Can you work these out from the model? Positions are in its coordinate system, mm. A direction names the side the tool comes from. Give positions to 0.01 mm unless a question says otherwise; leave off trailing zeros. Loops run counter-clockwise (first coordinate to the right, second up) from the corner with the lowest first, then second, coordinate; pieces in that order, holes last. Notation, with made-up numbers: (2.5, 51) - (42.5, 51) arc R13 ccw to (42.5, 73) - close; hole circle Ø8 at (13, 68.25). An arc over 180 degrees is marked (long way). Use a Markdown table: item, result. Add a question column.
Autodesk Inventor part; units mm, degrees
ref_plane "YZ Plane" through (0, 0, 0) normal (1, 0, 0) x (0, 1, 0)
ref_plane "XZ Plane" through (0, 0, 0) normal (0, 1, 0) x (-1, 0, 0)
ref_plane "XY Plane" through (0, 0, 0) normal (0, 0, 1) x (1, 0, 0)
sketch "Sketch1" plane through (0, 0, 0) normal (0, 1, 0) x (-1, 0, 0)
  line L0 (0, 0) -> (-380, 0)
  line L1 (-380, 0) -> (-380, -640)
  line L2 (-380, -640) -> (0, -640)
  line L3 (0, -640) -> (0, 0)
  dimension "d0" = 380
  dimension "d1" = 640
extrude "Extrusion1" add sketch "Sketch1" along normal blind 25
sketch "Sketch2" plane through (0, 25, 0) normal (0, 1, 0) x (1, 0, 0)
  line L0 (85, 120) -> (295, 120)
  line L1 (295, 120) -> (295, 520)
  line L2 (295, 520) -> (85, 520)
  line L3 (85, 520) -> (85, 120)
  line L4 (0, 640) -> (0, 0)
  line L5 (380, 640) -> (0, 640)
  dimension "d4" = 210
  dimension "d5" = 400
  dimension "d6" = 85
  dimension "d7" = 120
extrude "Extrusion2" add sketch "Sketch2" along normal blind 30
properties part number "Monitor, back bump not measured"
1. Suppose I cut it at D-D (z = -40). List the corners of the cut face in (x, y) for me, and give its area (3 significant figures).
2. Please list where these lines run through material, in increasing order: line 1 along Z through (x, y) = (142, 30.5); line 2 along X through (y, z) = (47.5, -153); line 3 along Y through (x, z) = (158, -118). Write a range as [from, to].
3. Suppose I cut it at B-B (x = 246.5). List the corners of the cut face in (y, z) for me, and give its area (3 significant figures).
4. Suppose I cut it at A-A (z = -257). List the corners of the cut face in (x, y) for me.
5. Suppose I cut it at C-C (y = 48.5). List the corners of the cut face in (x, z) for me.
6. Will these pins go through, and if not, where does the flat tip stop? P1, Ø24, axis at x = 195.5, y = 35.5, coming from the +Z side; P2, Ø12, axis at y = 43.5, z = -516.5, coming from the +X side; P3, Ø15, axis at x = 231.5, y = 39.5, coming from the -Z side; P4, Ø1, axis at y = 48.5, z = -257.5, coming from the -X side.
7. On a 3-axis mill with a long thin cutter (end or side, diameter ignored), from which of +Z, -Z, +X, -X, +Y, -Y can I reach the whole of each face in a straight line? I mean faces 1 (the face through (295, 40, -317)), 2 (the face through (191, 40, -520)), 3 (the face through (193, 12, -640)), 4 (the face through (189, 40, -120)), 5 (the face through (85, 40, -323)). Say none if no direction works.
Results below:
| question | item | result |
|---|---|---|
| 1 | outline | (0, 0) - (380, 0) - (380, 25) - (0, 25) - close |
| 1 | area | 9,500 mm² |
| 2 | line 1 | [-520, -120] |
| 2 | line 2 | [85, 295] |
| 2 | line 3 | [0, 25] |
| 3 | outline | (0, -640) - (25, -640) - (25, -520) - (55, -520) - (55, -120) - (25, -120) - (25, 0) - (0, 0) - close |
| 3 | area | 28,000 mm² |
| 4 | outline | (0, 0) - (380, 0) - (380, 25) - (295, 25) - (295, 55) - (85, 55) - (85, 25) - (0, 25) - close |
| 5 | outline | (85, -520) - (295, -520) - (295, -120) - (85, -120) - close |
| 6 | P1 | z = 0 |
| 6 | P2 | x = 295 |
| 6 | P3 | z = -520 |
| 6 | P4 | x = 85 |
| 7 | face 1 | +Z, -Z, +X, +Y |
| 7 | face 2 | -Z, +X, -X, +Y |
| 7 | face 3 | -Z, +X, -X, +Y, -Y |
| 7 | face 4 | +Z, +X, -X, +Y |
| 7 | face 5 | +Z, -Z, -X, +Y |
